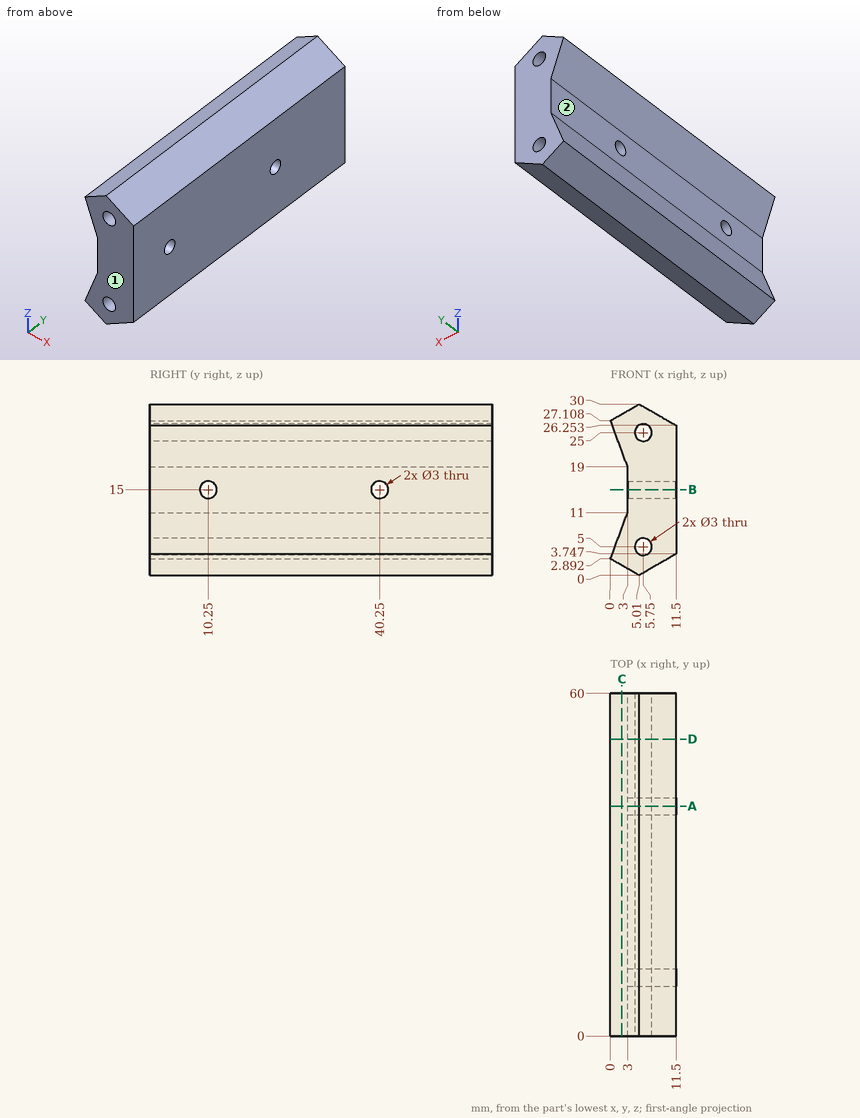
Geometry check sheet. Reference: drawing and pictorial views, mm from the part's lowest x, y, z. A direction names the side the tool comes from. Coordinates: 2 decimals unless noted, no trailing zeros. Order: outer loops, then holes, each group sorted by start corner. A loop starts at its lowest first (then second) coordinate and runs counter-clockwise, first axis right, second up.
Item 1: Tool access check on the marked faces 1 and 2. Record the directions out of +Z, -Z, +X, -X, +Y, -Y that give a thin tool (end or side, any length) a straight path to the whole face; none if there is none.
Item 2: Section check A-A (y = 40.25). Enter the section's corners in (x, z).
Item 3: Depth check by flat-ended pin: pin 1 (1 mm diameter, centred on x = 8.5, y = 28.5, fed in from -Z); pin 2 (2.5 mm diameter, centred on y = 31, z = 13.5, fed in from -X); pin 3 (10 mm diameter, centred on y = 51.5, z = 20, fed in from -X). Enter the tip coordinate at first touch or a pass-through.
Item 4: Section check B-B (z = 15). Enter the section's corners in (x, y), plus the area to 3 significant figures.
Item 5: Scan lines: line 1 along Z through (x, y) = (5.75, 33); line 2 along X through (y, z) = (36.5, 11.5); line 3 along Y through (x, z) = (9.5, 15.75). Record each from-to range of solid material in increasing order.
Item 6: Section check C-C (x = 2). Enter the section's corners in (y, z), plus the area to 3 significant figures.
Item 7: Section check D-D (y = 52). Enter the section's corners in (x, z).
Check sheet entries:
1. face 1: +Z, -Z, +X, -X, -Y
1. face 2: -X, +Y, -Y
2. outline: (0, 2.89) - (5.01, 0) - (11.5, 3.75) - (11.5, 13.5) - (3, 13.5) - (3, 11) - close; (0, 27.11) - (3, 19) - (3, 16.5) - (11.5, 16.5) - (11.5, 26.25) - (5.01, 30) - close; hole circle Ø3 at (5.75, 5); hole circle Ø3 at (5.75, 25)
3. pin 1: stops at z = 1.73
3. pin 2: stops at x = 3
3. pin 3: stops at x = 0.78
4. outline: (3, 0) - (11.5, 0) - (11.5, 8.75) - (3, 8.75) - close; (3, 11.75) - (11.5, 11.75) - (11.5, 38.75) - (3, 38.75) - close; (3, 41.75) - (11.5, 41.75) - (11.5, 60) - (3, 60) - close
4. area: 459 mm2
5. line 1: z = 0.43 to 3.5, 6.5 to 23.5, 26.5 to 29.57
5. line 2: x = 3 to 11.5
5. line 3: y = 0 to 8.95, 11.55 to 38.95, 41.55 to 60
6. outline: (0, 1.74) - (60, 1.74) - (60, 8.3) - (0, 8.3) - close; (0, 21.7) - (60, 21.7) - (60, 28.26) - (0, 28.26) - close
6. area: 787 mm2
7. outline: (0, 2.89) - (5.01, 0) - (11.5, 3.75) - (11.5, 26.25) - (5.01, 30) - (0, 27.11) - (3, 19) - (3, 11) - close; hole circle Ø3 at (5.75, 5); hole circle Ø3 at (5.75, 25)
